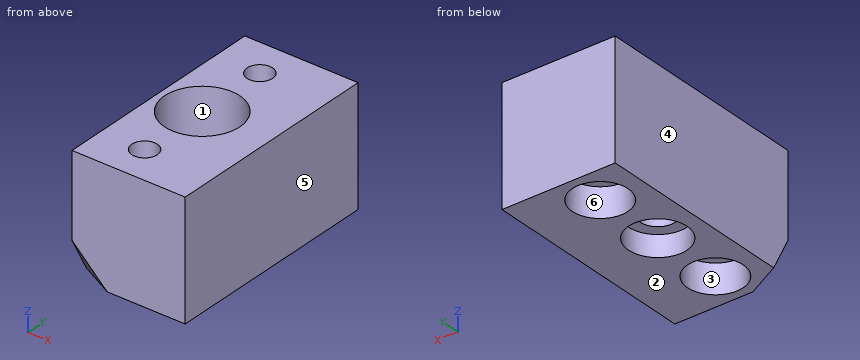
from build123d import *

# Parameters (mm, degrees)
SKETCH1_W               = 19
SKETCH1_H               = 30
BOSS_EXTRUDE1_DEPTH     = 18
SKETCH2_R               = 5.159375
CUT_EXTRUDE1_DEPTH      = 11.5
SKETCH4_R               = 4.8
CUT_EXTRUDE3_DEPTH      = 0.5
SKETCH5_R               = 2.38125
CUT_EXTRUDE4_DEPTH      = 13
CUT_EXTRUDE4_DEPTH_BACK = 8
CUT_EXTRUDE6_DEPTH      = 19
CUT_EXTRUDE6_DEPTH_BACK = 1
SKETCH11_W              = 15.5
SKETCH11_H              = 30
BOSS_EXTRUDE5_DEPTH     = 5
SKETCH12_R              = 4
CUT_EXTRUDE8_DEPTH      = 7.9
SKETCH13_R              = 1.75
CUT_EXTRUDE9_DEPTH      = 24
SKETCH15_W              = 15.5
SKETCH15_H              = 2
SKETCH15_H_2            = 5
CUT_EXTRUDE11_DEPTH     = 41
SKETCH17_R              = 5
CUT_EXTRUDE12_DEPTH     = 2
SKETCH20_R              = 3.81
CUT_EXTRUDE13_DEPTH     = 4


with BuildPart() as part:
    # Sketch1 → Boss-Extrude1 (new body)
    with BuildSketch(Plane.XY):
        Rectangle(SKETCH1_W, SKETCH1_H)
    extrude(amount=BOSS_EXTRUDE1_DEPTH)

    # Sketch2 → Cut-Extrude1 (cut)
    with BuildSketch(Plane.XY.offset(18)):
        Circle(SKETCH2_R)
    extrude(amount=-CUT_EXTRUDE1_DEPTH, mode=Mode.SUBTRACT)

    # Sketch4 → Cut-Extrude3 (cut)
    with BuildSketch(Plane.XY.offset(6.5)):
        Circle(SKETCH4_R)
    extrude(amount=-CUT_EXTRUDE3_DEPTH, mode=Mode.SUBTRACT)

    # Sketch5 → Cut-Extrude4 (cut, two sides)
    with BuildSketch(Plane.XY.offset(6)) as cut_extrude4_sk:
        Circle(SKETCH5_R)
    extrude(amount=CUT_EXTRUDE4_DEPTH, mode=Mode.SUBTRACT)
    extrude(cut_extrude4_sk.sketch, amount=-CUT_EXTRUDE4_DEPTH_BACK, mode=Mode.SUBTRACT)

    # Sketch6 → Cut-Extrude6 (cut, two sides)
    with BuildSketch(Plane.XY) as cut_extrude6_sk:
        Polygon((-6, 92.53517602), (-6, 15), (-6, -15), (-6, -92.53517602), (-161.070352039, -92.53517602), (-161.070352039, 92.53517602), align=None)
    extrude(amount=CUT_EXTRUDE6_DEPTH, mode=Mode.SUBTRACT)
    extrude(cut_extrude6_sk.sketch, amount=-CUT_EXTRUDE6_DEPTH_BACK, mode=Mode.SUBTRACT)

    # Sketch11 → Boss-Extrude5 (add)
    with BuildSketch(Plane(origin=(0, 0, 0), x_dir=(-1, 0, 0), z_dir=(0, 0, -1))):
        with Locations((-1.75, 0)):
            Rectangle(SKETCH11_W, SKETCH11_H)
    extrude(amount=BOSS_EXTRUDE5_DEPTH)

    # Sketch12 → Cut-Extrude8 (cut)
    with BuildSketch(Plane(origin=(0, 0, -5), x_dir=(-1, 0, 0), z_dir=(0, 0, -1))):
        Circle(SKETCH12_R)
    extrude(amount=-CUT_EXTRUDE8_DEPTH, mode=Mode.SUBTRACT)

    # Sketch13 → Cut-Extrude9 (cut, through all)
    with BuildSketch(Plane(origin=(0, 0, -5), x_dir=(-1, 0, 0), z_dir=(0, 0, -1))):
        with Locations((0, -10)):
            Circle(SKETCH13_R)
        with Locations((0, 10)):
            Circle(SKETCH13_R)
    extrude(amount=-CUT_EXTRUDE9_DEPTH, mode=Mode.SUBTRACT)

    # Sketch15 → Cut-Extrude11 (cut)
    with BuildSketch(Plane.XZ.offset(15)):
        with Locations((1.75, 17)):
            Rectangle(SKETCH15_W, SKETCH15_H)
        with Locations((1.75, -2.5)):
            Rectangle(SKETCH15_W, SKETCH15_H_2)
    extrude(amount=-CUT_EXTRUDE11_DEPTH, mode=Mode.SUBTRACT)

    # Sketch17 → Cut-Extrude12 (cut)
    with BuildSketch(Plane(origin=(-6, -15, 0), x_dir=(0.909907666, -0.366009572, -0.195205105), z_dir=(0.414810848, 0.802859705, 0.428191843))):
        Circle(SKETCH17_R)
    extrude(amount=CUT_EXTRUDE12_DEPTH, mode=Mode.SUBTRACT)

    # Sketch20 → Cut-Extrude13 (cut)
    with BuildSketch(Plane(origin=(0, 0, 0), x_dir=(-1, 0, 0), z_dir=(0, 0, -1))):
        with Locations((0, 10)):
            Circle(SKETCH20_R)
        with Locations((0, -10)):
            Circle(SKETCH20_R)
    extrude(amount=-CUT_EXTRUDE13_DEPTH, mode=Mode.SUBTRACT)


solid = part.part
Part model, mm, in its own coordinate system. Face numbers are marked on the shaded views. A direction names the side the tool comes from. Give positions to 0.01 mm unless a question says otherwise; leave off trailing zeros. Loops run counter-clockwise (first coordinate to the right, second up) from the corner with the lowest first, then second, coordinate; pieces in that order, holes last. Notation, with made-up numbers: M -8,53.25 L 42,53.25 A20 cw 42,59.25 Z; hole C 9,-27.5 d11. An arc over 180 degrees is marked long. Put each result on its own line as item: value. Start each with the question number.
1) Probe probe 1 along Y at (x, z) = (0, 12.25); probe 2 along Y at (x, z) = (0, 6.3); probe 3 along Z at (x, y) = (-3.5, 10). List the from-to ranges inside material, lowest first.
2) 3-axis set-ups, long thin cutter, end or side, ignore diameter. For the marked faces 1, 2 and 3: which of +Z, -Z, +X, -X, +Y, -Y reach the whole face in a straight line?
3) Saw through at C-C (y = 9). List the corners of the cut face in (x, z).
4) Flat gauge pins, fed straight in: pin 1 (2.5 mm diameter, centred on x = 0.5, y = -8, fed in from -Z); pin 2 (7 mm diameter, centred on x = 0, y = 0, fed in from +Z); pin 3 (4 mm diameter, centred on x = 1, y = 1.5, fed in from -Z). Where does each tip first touch, or does it go through?
5) Saw through at B-B (z = 7.25). List the corners of the cut face in (x, y).
6) Pull direction X, two halves, no side cores. Call the marked faces 4, 5 and 6: +X half, -X half, draft (parallel to the pull), parting line (faces both ways), or undercut.
7) Saw through at D-D (x = -3.5). List the corners of the cut face in (y, z).
8) Saw through at A-A (y = -10). List the corners of the cut face in (x, z), then the cut area to 3 significant figures.
Numbers:
1. probe 1: -15 to -11.75, -8.25 to -5.16, 5.16 to 8.25, 11.75 to 15
1. probe 2: -15 to -11.75, -8.25 to -4.8, 4.8 to 8.25, 11.75 to 15
1. probe 3: 4 to 16
2. face 1: +Z
2. face 2: -Z, +X, -X, +Y, -Y
2. face 3: -Z
3. outline: M -6,0 L -3.68,0 L -3.68,4 L -1.44,4 L -1.44,16 L -6,16 Z; M 1.44,4 L 3.68,4 L 3.68,0 L 9.5,0 L 9.5,16 L 1.44,16 Z
4. pin 1: z = 4
4. pin 2: z = 6
4. pin 3: z = 2.9
5. outline: M -6,-15 L 9.5,-15 L 9.5,15 L -6,15 Z; hole C 0,0 d10.32; hole C 0,-10 d3.5; hole C 0,10 d3.5
6. face 4: -X half
6. face 5: +X half
6. face 6: undercut
7. outline: M -15,2.25 L -13.8,0 L -11.51,0 L -11.51,4 L -8.49,4 L -8.49,0 L -1.94,0 L -1.94,2.9 L 1.94,2.9 L 1.94,0 L 8.49,0 L 8.49,4 L 11.51,4 L 11.51,0 L 15,0 L 15,16 L 3.79,16 L 3.79,6.5 L 3.28,6.5 L 3.28,6 L -3.28,6 L -3.28,6.5 L -3.79,6.5 L -3.79,16 L -15,16 Z
8. outline: M -6,0 L -3.81,0 L -3.81,4 L -1.75,4 L -1.75,16 L -6,16 Z; M 1.75,4 L 3.81,4 L 3.81,0 L 9.5,0 L 9.5,16 L 1.75,16 Z
8. area: 176 mm^2
